from build123d import *
from OCP.BRepFilletAPI import BRepFilletAPI_MakeChamfer

# Parameters (mm, degrees)
SKICA1_W                = 84
SKICA1_H                = 84
P_IDAT_VYSUNUT_M1_DEPTH = 1.6
SKICA1_3_W              = 80
SKICA1_3_H              = 80
SKICA1_3_W_2            = 20
SKICA1_3_H_2            = 76.8
SKICA1_3_W_3            = 55.2
SKICA1_3_H_3            = 37.6
P_IDAT_VYSUNUT_M2_DEPTH = 14
SKICA1_4_W              = 84
SKICA1_4_H              = 84
SKICA1_4_W_2            = 80
SKICA1_4_H_2            = 80
P_IDAT_VYSUNUT_M3_DEPTH = 4
ZKOSEN_2_SIZE           = 3.464101615
ZKOSEN_2_SIZE_2         = 2


with BuildPart() as part:
    # Skica1 → Přidat vysunutím1 (new body)
    with BuildSketch(Plane(origin=(0, 0, 0), x_dir=(1, 0, 0), z_dir=(0, 1, 0))):
        with Locations((-42, 42)):
            Rectangle(SKICA1_W, SKICA1_H)
    extrude(amount=P_IDAT_VYSUNUT_M1_DEPTH)

    # Skica1<3> → Přidat vysunutím2 (add)
    with BuildSketch(Plane(origin=(0, 0, 0), x_dir=(1, 0, 0), z_dir=(0, 1, 0))):
        with Locations((-42, 42)):
            Rectangle(SKICA1_3_W, SKICA1_3_H)
        with Locations((-13.6, 42)):
            Rectangle(SKICA1_3_W_2, SKICA1_3_H_2, mode=Mode.SUBTRACT)
        with Locations((-52.8, 61.6)):
            Rectangle(SKICA1_3_W_3, SKICA1_3_H_3, mode=Mode.SUBTRACT)
        with Locations((-52.8, 22.4)):
            Rectangle(SKICA1_3_W_3, SKICA1_3_H_3, mode=Mode.SUBTRACT)
    extrude(amount=P_IDAT_VYSUNUT_M2_DEPTH)

    # Skica1<4> → Přidat vysunutím3 (add)
    with BuildSketch(Plane(origin=(0, 0, 0), x_dir=(1, 0, 0), z_dir=(0, 1, 0))):
        with Locations((-42, 42)):
            Rectangle(SKICA1_4_W, SKICA1_4_H)
        with Locations((-42, 42)):
            Rectangle(SKICA1_4_W_2, SKICA1_4_H_2, mode=Mode.SUBTRACT)
    extrude(amount=P_IDAT_VYSUNUT_M3_DEPTH)

    # Zkosení2
    zkosen_2_edges_1 = [part.edges().sort_by_distance(p)[0] for p in [
        (-84, 4, -42),
    ]]
    zkosen_2_side_1 = [part.faces().sort_by_distance(p)[0] for p in [
        (-84, 3.96, -42),
    ]]
    zkosen_2_edges_2 = [part.edges().sort_by_distance(p)[0] for p in [
        (-42, 4, 0),
    ]]
    zkosen_2_side_2 = [part.faces().sort_by_distance(p)[0] for p in [
        (-42, 3.96, 0),
    ]]
    zkosen_2_edges_3 = [part.edges().sort_by_distance(p)[0] for p in [
        (0, 4, -42),
    ]]
    zkosen_2_side_3 = [part.faces().sort_by_distance(p)[0] for p in [
        (-0.04, 4, -42),
    ]]
    zkosen_2_edges_4 = [part.edges().sort_by_distance(p)[0] for p in [
        (-42, 4, -84),
    ]]
    zkosen_2_side_4 = [part.faces().sort_by_distance(p)[0] for p in [
        (-42, 3.96, -84),
    ]]
    zkosen_2 = BRepFilletAPI_MakeChamfer(part.part.solid().wrapped)
    for e in zkosen_2_edges_1:
        zkosen_2.Add(ZKOSEN_2_SIZE - 0.0001, ZKOSEN_2_SIZE_2 - 0.0001, e.wrapped, zkosen_2_side_1[0].wrapped)
    for e in zkosen_2_edges_2:
        zkosen_2.Add(ZKOSEN_2_SIZE - 0.0001, ZKOSEN_2_SIZE_2 - 0.0001, e.wrapped, zkosen_2_side_2[0].wrapped)
    for e in zkosen_2_edges_3:
        zkosen_2.Add(ZKOSEN_2_SIZE_2 - 0.0001, ZKOSEN_2_SIZE - 0.0001, e.wrapped, zkosen_2_side_3[0].wrapped)
    for e in zkosen_2_edges_4:
        zkosen_2.Add(ZKOSEN_2_SIZE - 0.0001, ZKOSEN_2_SIZE_2 - 0.0001, e.wrapped, zkosen_2_side_4[0].wrapped)
    add(Compound.cast(zkosen_2.Shape()), mode=Mode.REPLACE)  # a hair under: the kernel refuses the full size


solid = part.part
Source: CAD feature listing. Evaluate the final solid. Frame: model axes, mm. A direction names the side the tool comes from. Give positions to 0.01 mm unless a question says otherwise; leave off trailing zeros. Write each loop counter-clockwise with the first axis right and the second up, starting at its lowest first coordinate (ties: lowest second). Pieces come first, ordered by that corner, then holes. Notation, with made-up numbers: M -10.5,53 L 39.5,53 A9 ccw 39.5,66 Z; hole C -35,13.25 d9. An arc over 180 degrees is marked long. Return JSON: item names as keys, results as strings. Group by question number.
1) Cut plane A-A, the plane y = 13. Output: boundary loops of the cut face in (x, z), plus the area to 3 significant figures.
2) Set-up query: faces 1 (the face through (-14, 8, -3.6)), 2 (the face through (-82, 9, -41)), 3 (the face through (-42.588, 2.292, -1.014)), 4 (the face through (-2, 9, -41)). Return all of +Z, -Z, +X, -X, +Y, -Y with unobstructed straight access to the full face (end or side cutting, diameter ignored); none if empty.
3) Pull-direction query (Z, two-part tool) for faces 5 (the face through (-14, 8, -80.4)), 6 (the face through (-43, 0, -43)), 7 (the face through (-43, 9, -2)); classes: pulls with the +Z half, pulls with the -Z half, needs draft (parallel to the pull), parting line crosses it, or undercut.
4) Material intervals for line 1 along X through (y, z) = (5.5, -59); line 2 along Z through (x, y) = (-43.5, 8.75); line 3 along X through (y, z) = (2, -50.5), sorted ascending. Write a range as [from, to].
5) Pin query (flat end, axial travel): P1, Ø4, axis at y = 10.5, z = -72.5, coming from the -X side; P2, Ø11.5, axis at x = -66, z = -64.5, coming from the +Y side; P3, Ø3, axis at x = -50, y = 2.5, coming from the +Z side; P4, Ø4, axis at x = -8.5, z = -42, coming from the -Y side. Return the tip coordinate at first contact, or that it passes through.
Recorded:
{
 "1": {"outline": "M -82,-82 L -2,-82 L -2,-2 L -82,-2 Z; hole M -80.4,-80.4 L -25.2,-80.4 L -25.2,-42.8 L -80.4,-42.8 Z; hole M -80.4,-41.2 L -25.2,-41.2 L -25.2,-3.6 L -80.4,-3.6 Z; hole M -23.6,-80.4 L -3.6,-80.4 L -3.6,-3.6 L -23.6,-3.6 Z", "area": "713 mm²"},
 "2": {"face 1": "+Y", "face 2": "+Z, -Z, -X, +Y", "face 3": "+Z, +X, -X, +Y", "face 4": "+Z, -Z, +X, +Y"},
 "3": {"face 5": "undercut", "face 6": "needs draft", "face 7": "pulls with the +Z half"},
 "4": {"line 1": "x = [-82, -80.4], [-25.2, -23.6], [-3.6, -2]", "line 2": "z = [-82, -80.4], [-42.8, -41.2], [-3.6, -2]", "line 3": "x = [-83.15, -80.4], [-25.2, -23.6], [-3.6, -0.85]"},
 "5": {"P1": "stops at x = -82", "P2": "stops at y = 1.6", "P3": "stops at z = -0.27", "P4": "stops at y = 0"}
}
